Model file for the job. Use its own axes, mm. A direction names the side the tool comes from. Give positions to 0.01 mm unless a question says otherwise; leave off trailing zeros. Loops run counter-clockwise (first coordinate to the right, second up) from the corner with the lowest first, then second, coordinate; pieces in that order, holes last. Notation, with made-up numbers: M -2.75,-29.75 L 13.25,-29.75 A28 ccw 13.25,-7.75 Z; hole C 71,-21 d4. An arc over 180 degrees is marked long. Use CSV: the item, a comma, the result in double quotes. Start each with the question number.
(1) Slice it at D-D on x = 1.75. List the corners of the cut face in (y, z).
(2) Two-plate mould, pull along Y, no slides. Class faces 4 (the face through (4.9, 1, 0)), 5 (the face through (0, 3, 0)), 6 (the face through (-2, -21, 7)), 7 (the face through (0, -9, 2.5)): pulls with the +Y half, pulls with the -Y half, needs draft (parallel to the pull), parting line crosses it, or undercut.
(3) Slice it at B-B on x = -0.75. List the corners of the cut face in (y, z).
(4) Wall check: line 1 along Y through (x, z) = (4, -3); line 2 along Z through (x, y) = (0, -7); line 3 along Z through (x, y) = (-0.5, 0.5). Give the ranges that are in metal, low to high. Write a range as from..to.
(5) Tool access for faces 1 (the face through (2.5, -13, 2)), 2 (the face through (-2, 0, -2)), 3 (the face through (1.748, -8.381, -1.787)): list every direction of +Z, -Z, +X, -X, +Y, -Y with a clear straight run to the whole face (end or side of a thin tool).
(6) Flat gauge pins, fed straight in: P1, Ø2, axis at x = 0.5, y = -7.5, coming from the +Z side; P2, Ø9.5, axis at y = -6, z = 4.5, coming from the +X side; P3, Ø0.9, axis at x = 2, y = 1.5, coming from the +Z side. Where does each tip first touch, or does it go through?
```python
from build123d import *

# Parameters (mm, degrees)
F0_W     = 9.8
F0_H     = 9.8
F2_DEPTH = 3
F1_W     = 17
F1_H     = 5
F3_DEPTH = 2.5
F4_R     = 2.49999


# Not quite as in the source:
# - a fillet or chamfer is up to 0.001 mm smaller than in the source, because OpenCascade refuses the exact size


with BuildPart() as f2:
    # F0 (on Front) → F2 (new body)
    with BuildSketch(Plane.XZ):
        Rectangle(F0_W, F0_H)
    extrude(amount=-F2_DEPTH)

    # F1 (on Right) → F3 (join, symmetric)
    with BuildSketch(Plane.YZ):
        with Locations((-8.5, 0)):
            Rectangle(F1_W, F1_H)
        Polygon((-17, -2.5), (-17, 2.5), (-17, 12), (-22, 12), (-22, 2.5), align=None)
    extrude(amount=F3_DEPTH, both=True)

    # F4 (radius 2.5 in the source; OpenCascade refuses exactly that, so slightly less here)
    f4_edges = [f2.edges().sort_by_distance(p)[0] for p in [
        (-2.5, -8.5, -2.5),
        (-2.5, -19.5, 0),
        (2.5, -8.5, -2.5),
        (2.5, -19.5, 0),
        (2.5, -22, 7.25),
        (-2.5, -22, 7.25),
    ]]
    fillet(f4_edges, radius=F4_R)


solid = f2.part
```
Reply:
1,outline,"M -21.29,2.8 L -16.7,-1.79 L 0,-1.79 L 0,-4.9 L 3,-4.9 L 3,4.9 L 0,4.9 L 0,2.5 L -17,2.5 L -17,12 L -21.29,12 Z"
2,face 4,"needs draft"
2,face 5,"pulls with the +Y half"
2,face 6,"pulls with the -Y half"
2,face 7,"undercut"
3,outline,"M -21.88,2.55 L -16.95,-2.38 L 0,-2.38 L 0,-4.9 L 3,-4.9 L 3,4.9 L 0,4.9 L 0,2.5 L -17,2.5 L -17,12 L -21.88,12 Z"
4,line 1,"y = 0..3"
4,line 2,"z = -2.5..2.5"
4,line 3,"z = -4.9..4.9"
5,face 1,"+Z, -Z, +X, -Y"
5,face 2,"none"
5,face 3,"-Z, +X, -Y"
6,P1,"stops at z = 2.5"
6,P2,"stops at x = 2.5"
6,P3,"stops at z = 4.9"
